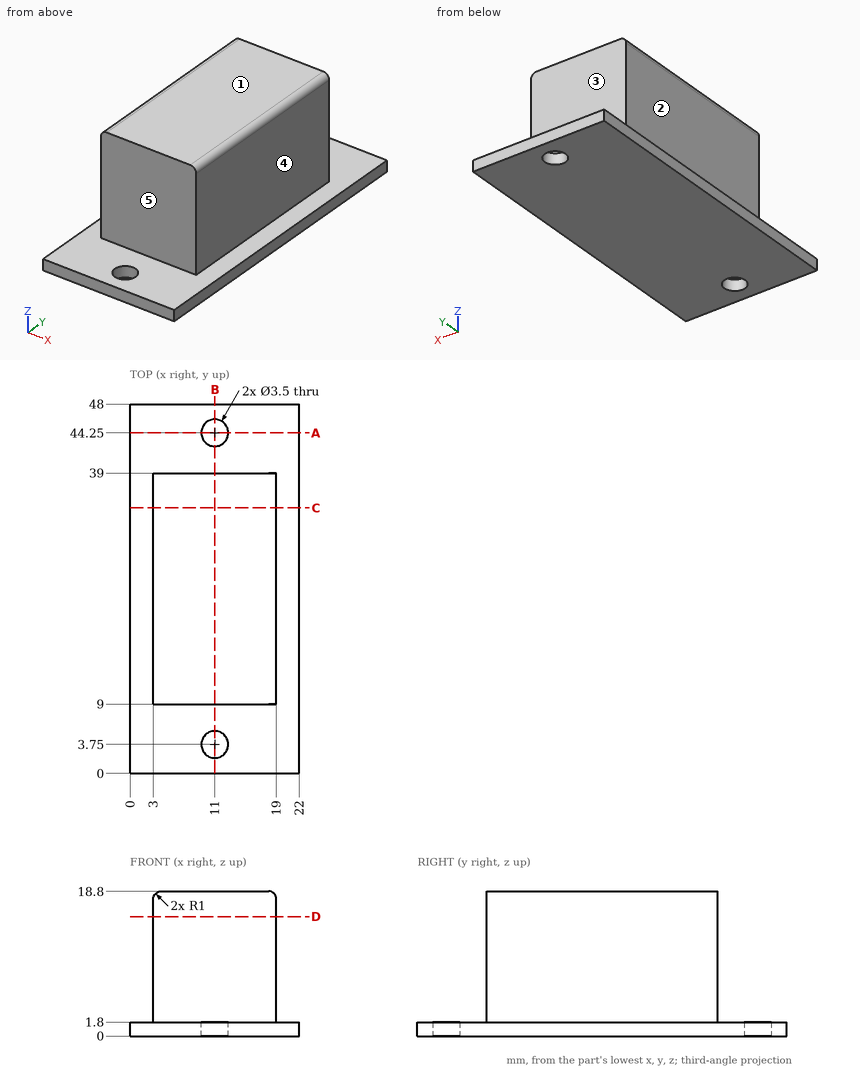
Part print with two shaded views. Sizes in mm from the minimum x, y, z corner. A direction names the side the tool comes from. Round coordinates to 2 decimals unless told otherwise and drop trailing zeros. Loops run counter-clockwise (first coordinate to the right, second up) from the corner with the lowest first, then second, coordinate; pieces in that order, holes last.
1. Slice it at C-C (y = 34.5). Give the cut face in (x, z).
Solutions:
outline: (0, 0) - (22, 0) - (22, 1.8) - (19, 1.8) - (19, 17.8) arc R1 ccw to (18, 18.8) - (4, 18.8) arc R1 ccw to (3, 17.8) - (3, 1.8) - (0, 1.8) - close
2. Slice it at D-D (z = 15.5). Give the cut face in (x, y).
Solutions:
outline: (3, 9) - (19, 9) - (19, 39) - (3, 39) - close
3. 3-axis set-ups, long thin cutter, end or side, ignore diameter. For the marked faces 1, 2, 3, 4 and 5: which of +Z, -Z, +X, -X, +Y, -Y reach the whole face in a straight line?
Solutions:
face 1: +Z, +X, -X, +Y, -Y
face 2: +Z, -X, +Y, -Y
face 3: +Z, +X, -X, +Y
face 4: +Z, +X, +Y, -Y
face 5: +Z, +X, -X, -Y
4. Drill centre lines: line 1 along Y through (x, z) = (11, 1.1); line 2 along Z through (x, y) = (19.75, 14); line 3 along Y through (x, z) = (10, 7.25). Where is each one in solid material? Low to high.
Solutions:
line 1: y = 0 to 2, 5.5 to 42.5, 46 to 48
line 2: z = 0 to 1.8
line 3: y = 9 to 39
5. Slice it at B-B (x = 11). Give the cut face in (y, z).
Solutions:
outline: (0, 0) - (2, 0) - (2, 1.8) - (0, 1.8) - close; (5.5, 0) - (42.5, 0) - (42.5, 1.8) - (39, 1.8) - (39, 18.8) - (9, 18.8) - (9, 1.8) - (5.5, 1.8) - close; (46, 0) - (48, 0) - (48, 1.8) - (46, 1.8) - close
6. Flat gauge pins, fed straight in: pin 1 (1.5 mm diameter, centred on x = 6, z = 11.5, fed in from +Y); pin 2 (8 mm diameter, centred on y = 23.5, z = 12.5, fed in from -X); pin 3 (4.5 mm diameter, centred on x = 11, y = 3.75, fed in from +Z). Where does each tip first touch, or does it go through?
Solutions:
pin 1: stops at y = 39
pin 2: stops at x = 3
pin 3: stops at z = 1.8
7. Slice it at A-A (y = 44.25). Give the cut face in (x, z).
Solutions:
outline: (0, 0) - (9.25, 0) - (9.25, 1.8) - (0, 1.8) - close; (12.75, 0) - (22, 0) - (22, 1.8) - (12.75, 1.8) - close
